Autodesk Inventor part; units mm, degrees
ref_plane "YZ Plane" through (0, 0, 0) normal (1, 0, 0) x (0, 1, 0)
ref_plane "XZ Plane" through (0, 0, 0) normal (0, 1, 0) x (-1, 0, 0)
ref_plane "XY Plane" through (0, 0, 0) normal (0, 0, 1) x (1, 0, 0)
sketch "Sketch1" plane through (0, 0, 0) normal (0, 0, 1) x (1, 0, 0)
  line L0 (0, 0) -> (90, 0)
  line L1 (90, 0) -> (90, 150)
  line L2 (90, 150) -> (0, 150)
  line L3 (0, 150) -> (0, 0)
  line L4 (90, 100) -> (59, 100)
  line L5 (59, 100) -> (59, 50)
  line L6 (59, 50) -> (90, 50)
  line L7 (90, 50) -> (90, 100)
  point P0 (-56.8499, 87.1082)
  dimension "d0" = 90
  dimension "d1" = 150
  dimension "d2" = 31
sketch "Sketch2" plane through (0, 0, 0) normal (0, 0, 1) x (1, 0, 0)
  point P0 (0, 0)
extrude "Extrusion1" add sketch "Sketch1" along normal blind 3 contours L3 L2 L1 L4 L5 L6 L0
properties part number "bridge plate"
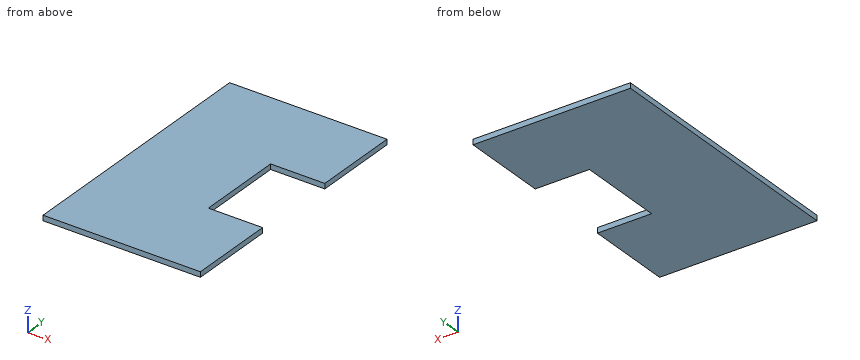
The model under review builds one solid part; all positions refer to its coordinate system, in mm. Round coordinates to 2 decimals unless told otherwise and drop trailing zeros. Loops run counter-clockwise (first coordinate to the right, second up) from the corner with the lowest first, then second, coordinate; pieces in that order, holes last. Notation, with made-up numbers: M 59.25,63.25 L 72.25,63.25 A14 ccw 72.25,84.25 Z; hole C -4.75,-6 d9. An arc over 180 degrees is marked long. Answer as CSV lines item,"result". Start each with the question number.
Item 1: Consider section A-A (x = 60.5). Write out the cut boundary in (y, z).
Item 2: Wall thickness on line 1 (Y direction, x = 82, z = 0.4); line 2 (X direction, y = 97, z = 1.05): over which ranges is each line inside the solid? List them lowest first. Write a range as [from, to].
Item 3: Consider section B-B (z = 1.15). Write out the cut boundary in (x, y), then the cut area to 4 significant figures.
Item 4: Consider section C-C (y = 61). Write out the cut boundary in (x, z).
Answer:
1,outline,"M 0,0 L 50,0 L 50,3 L 0,3 Z; M 100,0 L 150,0 L 150,3 L 100,3 Z"
2,line 1,"y = [0, 50], [100, 150]"
2,line 2,"x = [0, 59]"
3,outline,"M 0,0 L 90,0 L 90,50 L 59,50 L 59,100 L 90,100 L 90,150 L 0,150 Z"
3,area,"11,950 mm^2"
4,outline,"M 0,0 L 59,0 L 59,3 L 0,3 Z"
